Work out the finished part from the listing and answer in its coordinate system (mm). A direction names the side the tool comes from. Coordinates: 2 decimals unless noted, no trailing zeros. Order: outer loops, then holes, each group sorted by start corner. A loop starts at its lowest first (then second) coordinate and runs counter-clockwise, first axis right, second up. Notation, with made-up numbers: M 26.5,56 L 73.5,56 A18 cw 73.5,73 Z; hole C 53.25,65.25 d6. An arc over 180 degrees is marked long. Use a Markdown table: item, result.
Autodesk Fusion 360 part; units mm, degrees
sketch "Sketch1" plane through (0, 0, 0) normal (0, 1, 0) x (1, 0, 0)
  circle A0 centre (0, 0) radius 27.5
  circle A1 centre (0, 0) radius 10
  line L0 (0, 0) -> (13, 0)
  line L1 (0, 0) -> (0, 13)
  line L2 (0, 0) -> (-13, 0)
  line L3 (-13, 0) -> (-13, 1.55)
  line L4 (-13, 1.55) -> (-18, 1.55)
  line L5 (-13, 1.55) -> (-9.8791, 1.55)
  line L6 (-13, 0) -> (-13, -1.55)
  line L7 (-13, -1.55) -> (-9.8791, -1.55)
  line L8 (-13, -1.55) -> (-18, -1.55)
  line L9 (0, 13) -> (1.55, 13)
  line L10 (1.55, 13) -> (1.55, 18)
  line L11 (1.55, 18) -> (-1.55, 18)
  line L12 (-1.55, 18) -> (-1.55, 9.8791)
  line L13 (1.55, 9.8791) -> (1.55, 18)
  line L14 (13, 0) -> (13, -1.55)
  line L15 (13, -1.55) -> (18, -1.55)
  line L16 (18, -1.55) -> (9.8791, -1.55)
  line L17 (9.8791, 1.55) -> (18, 1.55)
  line L18 (18, 1.55) -> (18, -1.55)
  arc A2 (-18, 1.55) -> (-18, -1.55) centre (-18, 0) ccw
  arc A3 (1.55, 18) -> (-1.55, 18) centre (0, 18) ccw
  arc A4 (18, -1.55) -> (18, 1.55) centre (18, 0) ccw
  dimension "d12" = 13
  dimension "d13" = 13
  dimension "d14" = 13
  dimension "d15" = 1.55
  dimension "d16" = 5
  dimension "d17" = 1.55
  dimension "d18" = 1.55
  dimension "d19" = 5
  dimension "d20" = 3.1
  dimension "d21" = 1.55
  dimension "d22" = 5
  dimension "d23" = 3.1
extrude "Extrude1" add sketch "Sketch1" along normal blind 2
sketch "Sketch2" plane through (0, 2, 0) normal (0, 1, 0) x (-1, 0, 0)
  line L0 (-18, 1.55) -> (-9.8791, 1.55)
  arc A0 (9.8791, 1.55) -> (-9.8791, 1.55) centre (0, 0) ccw
  line L1 (9.8791, 1.55) -> (18, 1.55)
  arc A1 (18, -1.55) -> (18, 1.55) centre (18, 0) ccw
  line L2 (18, -1.55) -> (9.8791, -1.55)
  arc A2 (1.55, -9.8791) -> (9.8791, -1.55) centre (0, 0) ccw
  line L3 (1.55, -9.8791) -> (1.55, -18)
  arc A3 (-1.55, -18) -> (1.55, -18) centre (0, -18) ccw
  line L4 (-1.55, -18) -> (-1.55, -9.8791)
  arc A4 (-9.8791, -1.55) -> (-1.55, -9.8791) centre (0, 0) ccw
  line L5 (-9.8791, -1.55) -> (-18, -1.55)
  arc A5 (-18, 1.55) -> (-18, -1.55) centre (-18, 0) ccw
  circle A6 centre (0, 0) radius 27.5
  circle A7 centre (0, 0) radius 25.3
  circle A8 centre (0, 0) radius 22.5
  dimension "d26" = 50.6
  dimension "d27" = 45
extrude "Extrude2" add sketch "Sketch2" along normal blind 7 contours A7
ref_plane "WorkPlane2" through (25.5, 0, 0) normal (1, 0, 0) x (0, 1, 0)
sketch "Sketch4" plane through (25.5, 0, 0) normal (1, 0, 0) x (0, 0, -1)
  line L0 (0, 9) -> (0, 5.5)
  circle A0 centre (0, 5.5) radius 1.6
  point P0 (0, 9)
  dimension "d35" = 3.5
  dimension "d36" = 3.2
extrude "Extrude4" cut sketch "Sketch4" against normal through all
ref_plane "WorkPlane3" through (22.5, 0, 0) normal (1, 0, 0) x (0, 1, 0)
sketch "Sketch5" plane through (22.5, 0, 0) normal (1, 0, 0) x (0, 0, -1)
  line L0 (-1.7321, 8.5) -> (-3.4641, 5.5)
  line L1 (-3.4641, 5.5) -> (-1.7321, 2.5)
  line L2 (-1.7321, 2.5) -> (1.7321, 2.5)
  line L3 (1.7321, 2.5) -> (3.4641, 5.5)
  line L4 (3.4641, 5.5) -> (1.7321, 8.5)
  line L5 (1.7321, 8.5) -> (-1.7321, 8.5)
  point P0 (0, 5.5)
extrude "Extrude5" cut sketch "Sketch5" along normal blind 2 and the other way blind 1
pattern_circular "C-Pattern1" count 2 over 360 about axis through (0, 1.75, 0) along (0, 1, 0) of "Extrude5"
sketch "Sketch6" plane through (0, 0, 0) normal (1, 0, 0) x (0, 0, -1)
  line L0 (0, 9) -> (-2, 9)
  line L1 (1.55, 2) -> (9.8791, 2)
  line L2 (27.5, 2) -> (-27.5, 2)
  line L3 (28, 9) -> (28, 2)
  line L4 (28, 2) -> (-25.7716, 2)
  line L5 (-25.7716, 2) -> (-25.7716, 9)
  line L6 (0, 9) -> (-5, 9)
  line L7 (0, 9) -> (5, 9)
  line L8 (5, 9) -> (12, 2)
  line L9 (5, 9) -> (14.8995, 9) construction
  line L10 (-5, 9) -> (-12, 2)
  line L11 (28, 9) -> (-26, 9)
  point P0 (0, 9)
  dimension "d46" = 2
  dimension "d52" = 5
  dimension "d53" = 5
  dimension "d54" = 45
extrude "Extrude8" cut sketch "Sketch6" along normal mid plane 57.44 contours L2 L3 L4 L8 L11 | L2 L4 L5 L10 L11
(1) A cutting plane is placed at C-C (z = -13). Determine the outline of the cut face in (x, y).
Conclusion:
| item | result |
|---|---|
| outline | M -24.23,0 L -1.55,0 L -1.55,2 L -24.23,2 Z; M 1.55,0 L 24.23,0 L 24.23,2 L 1.55,2 Z |
(2) Which of the six approach directions +Z, -Z, +X, -X, +Y, -Y give full straight-line access (tool end or side, diameter ignored) to faces 4 (the flat face through (-1.55, 1, -14)), 5 (the flat face through (23, 2.5, 0)), 6 (the cylindrical face through (-25.3, 3.1, 0.2))?
Conclusion:
| item | result |
|---|---|
| face 4 | +Y, -Y |
| face 5 | none |
| face 6 | -X, +Y |
(3) A cutting plane is placed at A-A (z = 0). Give the number of separate pieces and of enclosed holes in the cut face, then the cut area to 3 significant figures.
Conclusion:
| item | result |
|---|---|
| separate pieces | 4 |
| enclosed holes | 0 |
| area | 41.9 mm2 |
(4) Straight lines are drawn through the part: L1, parallel to Y at x = 25.15, z = 0; L2, parallel to Y at x = -25, z = -6; L3, parallel to Y at x = -24, z = 0. For each, find the intervals that lie inside material, in ascending order.
Conclusion:
| item | result |
|---|---|
| L1 | 0 to 3.9, 7.1 to 9 |
| L2 | 0 to 2 |
| L3 | 0 to 2.5, 8.5 to 9 |
(5) A cutting plane is placed at B-B (x = -15). Determine the outline of the cut face in (y, z), then the cut area to 3 significant figures.
Conclusion:
| item | result |
|---|---|
| outline | M 0,-23.05 L 2,-23.05 L 2,-1.55 L 0,-1.55 Z; M 0,1.55 L 2,1.55 L 2,23.05 L 0,23.05 Z |
| area | 86.0 mm2 |
(6) Determine the mould class of faces 1 (the flat face through (24, 9, 0)), 2 (the flat face through (-23.3, 4, 2.6)), 3 (the flat face through (0, 0, 12)) for opening direction Y: pulls with the +Y half, pulls with the -Y half, needs draft (parallel to the pull), parting line crosses it, or undercut.
Conclusion:
| item | result |
|---|---|
| face 1 | pulls with the +Y half |
| face 2 | undercut |
| face 3 | pulls with the -Y half |
(7) Given P1, Ø1, axis at y = 1, z = -12, coming from the +X side; P2, Ø5, axis at y = 5.5, z = 0, coming from the +X side; P3, Ø1, axis at x = -4, z = -8.5, coming from the -Y side; P4, Ø2, axis at x = 12.5, y = 1, coming from the +Z side, each flat-ended and moving along its own axis, determine where each tip first touches the part or whether it passes through.
Conclusion:
| item | result |
|---|---|
| P1 | x = 24.98 |
| P2 | x = 25.3 |
| P3 | through |
| P4 | z = 24.98 |
(8) A cutting plane is placed at D-D (z = -7.5). Determine the outline of the cut face in (x, y).
Conclusion:
| item | result |
|---|---|
| outline | M -26.46,0 L -6.61,0 L -6.61,2 L -21.21,2 L -21.21,6.5 L -24.16,6.5 L -24.16,2 L -26.46,2 Z; M 6.61,0 L 26.46,0 L 26.46,2 L 24.16,2 L 24.16,6.5 L 21.21,6.5 L 21.21,2 L 6.61,2 Z |
